Part print with two shaded views. Sizes in mm from the minimum x, y, z corner. A direction names the side the tool comes from. Coordinates: 2 decimals unless noted, no trailing zeros. Order: outer loops, then holes, each group sorted by start corner. A loop starts at its lowest first (then second) coordinate and runs counter-clockwise, first axis right, second up. Notation, with made-up numbers: (70, 49) - (101, 49) arc R20 cw to (101, 63) - close; hole circle Ø6 at (-25, 5.5). An arc over 180 degrees is marked (long way). Return JSON: item names as keys, results as strings.
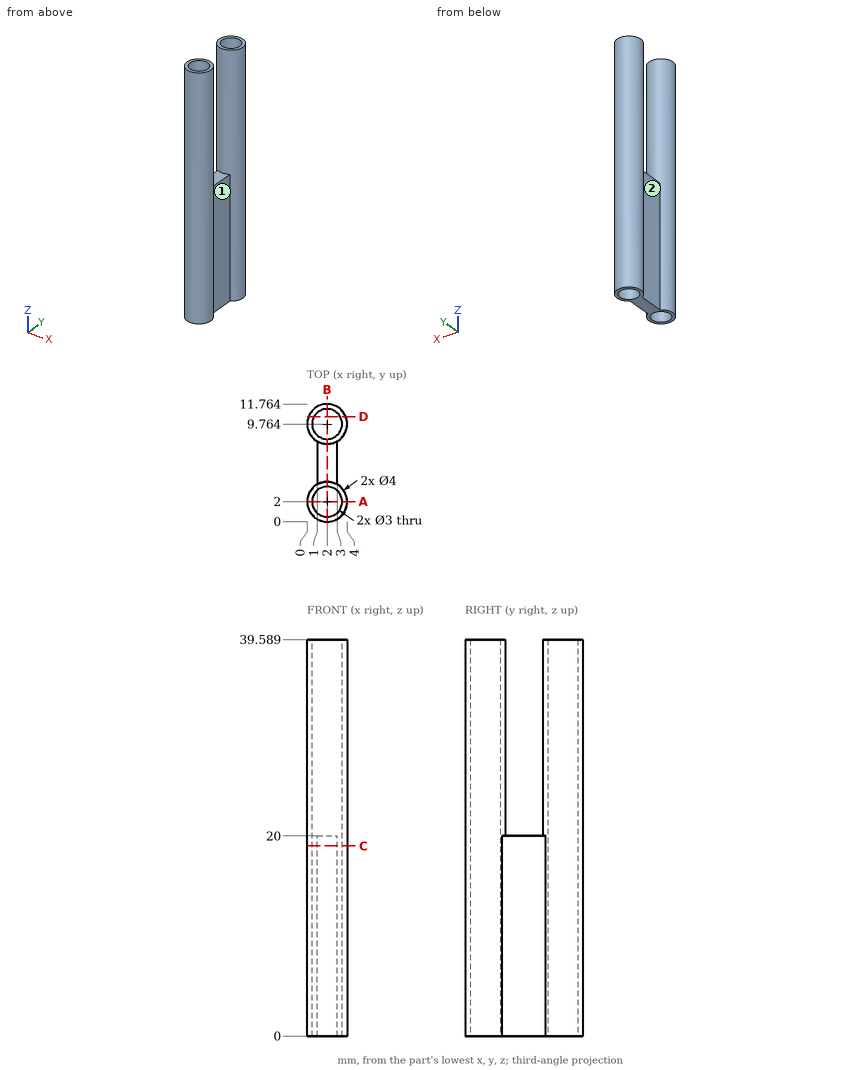
Item 1: Band-saw the part on C-C, the plane z = 19. List the corners of the cut face in (x, y) (1 decimal).
Findings below:
{"outline": "(1, 3.7) arc R2 ccw (long way) to (3, 3.7) - (3, 8) arc R2 ccw (long way) to (1, 8) - close; hole circle Ø3 at (2, 2); hole circle Ø3 at (2, 9.8)"}
Item 2: Band-saw the part on B-B, the plane x = 2. List the corners of the cut face in (y, z) (1 decimal).
Findings below:
{"outline": "(0, 0) - (0.5, 0) - (0.5, 39.6) - (0, 39.6) - close; (3.5, 0) - (8.3, 0) - (8.3, 39.6) - (7.8, 39.6) - (7.8, 20) - (4, 20) - (4, 39.6) - (3.5, 39.6) - close; (11.3, 0) - (11.8, 0) - (11.8, 39.6) - (11.3, 39.6) - close"}
Item 3: Which spindle directions (+Z, -Z, +X, -X, +Y, -Y) get a long thin tool onto all of the face, cutting with end or side? Do the marked faces 1 and 2. Say none if no direction does.
Findings below:
{"face 1": "+Z, -Z, +X", "face 2": "+Z, -Z, -X"}
Item 4: Drop flat-ended pins along their axis: P1, Ø1, axis at y = 8.5, z = 7, coming from the +X side; P2, Ø1.3, axis at y = 5.5, z = 13, coming from the +X side; P3, Ø2, axis at y = 7, z = 8, coming from the -X side. Give the stop position or say it passes through.
Findings below:
{"P1": "stops at x = 3.85", "P2": "stops at x = 3", "P3": "stops at x = 1"}
Item 5: Wall check: L1, parallel to Y at x = 2, z = 30.5 (1 decimal); L2, parallel to Y at x = 2, z = 18.5 (1 decimal); L3, parallel to Y at x = 2.7, z = 8 (1 decimal). Give the ranges that are in metal, low to high. Write a range as [from, to].
Findings below:
{"L1": "y = [0, 0.5], [3.5, 4], [7.8, 8.3], [11.3, 11.8]", "L2": "y = [0, 0.5], [3.5, 8.3], [11.3, 11.8]", "L3": "y = [0.1, 0.7], [3.3, 8.4], [11.1, 11.6]"}
Item 6: Band-saw the part on D-D, the plane y = 10.5. List the corners of the cut face in (x, z).
Findings below:
{"outline": "(0.14, 0) - (0.69, 0) - (0.69, 39.59) - (0.14, 39.59) - close; (3.31, 0) - (3.86, 0) - (3.86, 39.59) - (3.31, 39.59) - close"}
Item 7: Band-saw the part on A-A, the plane y = 2. List the corners of the cut face in (x, z).
Findings below:
{"outline": "(0, 0) - (0.5, 0) - (0.5, 39.59) - (0, 39.59) - close; (3.5, 0) - (4, 0) - (4, 39.59) - (3.5, 39.59) - close"}
